Part model, mm, in its own coordinate system. A direction names the side the tool comes from. Give positions to 0.01 mm unless a question says otherwise; leave off trailing zeros. Order: outer loops, then holes, each group sorted by start corner. A loop starts at its lowest first (then second) coordinate and runs counter-clockwise, first axis right, second up.
from build123d import *

# Parameters (mm, degrees)
F0_R     = 26.75
F1_DEPTH = 1.6
F2_R     = 26.75
F2_R_2   = 23.75
F3_DEPTH = 3
F4_R     = 26.75
F4_R_2   = 25.3
F5_DEPTH = 3
F6_R     = 6
F7_DEPTH = 25
F8_R     = 1.5
F9_DEPTH = 5


with BuildPart() as f1:
    # F0 (on Top) → F1 (new body)
    with BuildSketch(Plane.XY):
        Circle(F0_R)
    extrude(amount=F1_DEPTH)

    # F2 (on face) → F3 (join)
    with BuildSketch(Plane.XY.offset(1.6)):
        Circle(F2_R)
        Circle(F2_R_2, mode=Mode.SUBTRACT)
    extrude(amount=F3_DEPTH)

    # F4 (on face) → F5 (join)
    with BuildSketch(Plane.XY.offset(4.6)):
        Circle(F4_R)
        Circle(F4_R_2, mode=Mode.SUBTRACT)
    extrude(amount=F5_DEPTH)

    # F6 (on face) → F7 (cut)
    with BuildSketch(Plane.XY.offset(1.6)):
        Circle(F6_R)
    extrude(amount=-F7_DEPTH, mode=Mode.SUBTRACT)

    # F8 (on Top) → F9 (join)
    with BuildSketch(Plane.XY):
        with BuildLine():
            ThreePointArc((-26.40625, -4.2746299182), (-26.75, 0), (-26.40625, 4.2746299182))
            ThreePointArc((-26.40625, 4.2746299182), (-34, 0), (-26.40625, -4.2746299182))
        make_face()
        with Locations((-29, 0)):
            Circle(F8_R, mode=Mode.SUBTRACT)
        with BuildLine():
            ThreePointArc((26.40625, -4.2746299182), (31.4526771088, -4.3571062645), (34, 0))
            ThreePointArc((34, 0), (31.4526771088, 4.3571062645), (26.40625, 4.2746299182))
            ThreePointArc((26.40625, 4.2746299182), (26.6639240126, 2.1442145998), (26.75, 0))
            ThreePointArc((26.75, 0), (26.6639240126, -2.1442145998), (26.40625, -4.2746299182))
        make_face()
        with Locations((29, 0)):
            Circle(F8_R, mode=Mode.SUBTRACT)
    extrude(amount=F9_DEPTH)


solid = f1.part
Item 1: Pull direction X, two halves, no side cores. Call faces 3 (the face through (31, 0, 5)), 4 (the face through (-30.5, 0.07, 2.46)): released by +X, released by -X, zero draft, split by the parting line, or undercut.
Item 2: Drop flat-ended pins along their axis: P1, Ø2.5, axis at x = -29, y = -0.5, coming from the +Z side; P2, Ø1, axis at y = -15.5, z = 1.5, coming from the -X side; P3, Ø4, axis at y = 11.5, z = 1, coming from the -X side. Give the stop position or say it passes through.
Item 3: Drill centre lines: probe 1 along Y at (x, z) = (0, 6.8); probe 2 along Y at (x, z) = (0, 0.7); probe 3 along Z at (x, y) = (17, 14.5). Where is each one in solid material? Low to high.
Item 4: Band-saw the part on D-D on x = 0. List the corners of the cut face in (y, z), plus the area to 3 significant figures.
Item 5: Band-saw the part on C-C on y = 8.5. List the corners of the cut face in (x, z).
Item 6: Which spindle directions (+Z, -Z, +X, -X, +Y, -Y) get a long thin tool onto all of the face, cutting with end or side? Do faces 1 (the face through (27.5, 0.07, 2.46)), 2 (the face through (7, 23, 4.6)). Say none if no direction does.
Item 7: Band-saw the part on B-B on z = 6. List the corners of the cut face in (x, y).
Item 8: Band-saw the part on A-A on x = -29. List the corners of the cut face in (y, z).
Working result:
1. face 3: zero draft
1. face 4: undercut
2. P1: stops at z = 5
2. P2: stops at x = -22.15
2. P3: stops at x = -25.01
3. probe 1: y = -26.75 to -25.3, 25.3 to 26.75
3. probe 2: y = -26.75 to -6, 6 to 26.75
3. probe 3: z = 0 to 1.6
4. outline: (-26.75, 0) - (-6, 0) - (-6, 1.6) - (-23.75, 1.6) - (-23.75, 4.6) - (-25.3, 4.6) - (-25.3, 7.6) - (-26.75, 7.6) - close; (6, 0) - (26.75, 0) - (26.75, 7.6) - (25.3, 7.6) - (25.3, 4.6) - (23.75, 4.6) - (23.75, 1.6) - (6, 1.6) - close
4. area: 93.1 mm2
5. outline: (-25.36, 0) - (25.36, 0) - (25.36, 7.6) - (23.83, 7.6) - (23.83, 4.6) - (22.18, 4.6) - (22.18, 1.6) - (-22.18, 1.6) - (-22.18, 4.6) - (-23.83, 4.6) - (-23.83, 7.6) - (-25.36, 7.6) - close
6. face 1: +Z, -Z
6. face 2: +Z
7. outline: circle Ø53.5 at (0, 0); hole circle Ø50.6 at (0, 0)
8. outline: (-5, 0) - (-1.5, 0) - (-1.5, 5) - (-5, 5) - close; (1.5, 0) - (5, 0) - (5, 5) - (1.5, 5) - close
